CAD build for the part. Positions are in the model's coordinates, mm. A direction names the side the tool comes from. Give positions to 0.01 mm unless a question says otherwise; leave off trailing zeros. Write each loop counter-clockwise with the first axis right and the second up, starting at its lowest first coordinate (ties: lowest second). Pieces come first, ordered by that corner, then holes. Notation, with made-up numbers: (76, 29) - (95, 29) arc R20 ccw to (95, 57) - close; hole circle Ø6 at (-15, 77.25). An arc over 180 degrees is marked (long way). Answer as a JSON object with one key per item and string values.
from build123d import *

# Parameters (mm, degrees)
CUT_EXTRUDE1_DEPTH = 6
CUT_EXTRUDE2_DEPTH = 40


with BuildPart() as part:
    # Sketch1 → Revolve1 (revolve)
    with BuildSketch(Plane.XY):
        with BuildLine():
            Line((8.054036255, 0), (0, 4.65))
            Line((0, 4.65), (0, 11.233))
            Line((0, 11.233), (0.767, 12))
            Line((0.767, 12), (16.233, 12))
            Line((16.233, 12), (17.020818174, 11.212181826))
            ThreePointArc((17.020818174, 11.212181826), (19.144285046, 9.505211333), (21, 11.5))
            Line((21, 11.5), (21, 12.25))
            Line((21, 12.25), (30.021033995, 12.62983301))
            ThreePointArc((30.021033995, 12.62983301), (30.360913423, 12.783353536), (30.5, 13.129390385))
            Line((30.5, 13.129390385), (30.5, 13.175))
            Line((30.5, 13.175), (40, 13.65))
            Line((40, 13.65), (40, 0))
            Line((40, 0), (8.054036255, 0))
        make_face()
    revolve(axis=Axis((40, 0, 0), (-1, 0, 0)))

    # Sketch2 → Cut-Extrude1 (cut)
    with BuildSketch(Plane(origin=(0, 0, 0), x_dir=(0, 0, -1), z_dir=(1, 0, 0))):
        Polygon((-4, -2.309401077), (0, -4.618802154), (4, -2.309401077), (4, 2.309401077), (0, 4.618802154), (-4, 2.309401077), align=None)
    extrude(amount=CUT_EXTRUDE1_DEPTH, mode=Mode.SUBTRACT)

    # Sketch3 → Cut-Revolve1 (revolve, cut)
    with BuildSketch(Plane(origin=(0, 0, 0), x_dir=(1, 0, 0), z_dir=(0, 1, 0))):
        Polygon((6, 0), (6, 4.75), (8, 4.75), (8, 3.5), (10, 3.5), (10, 7.2), (12, 7.2), (12, 7), (42, 7), (42, 0), align=None)
    revolve(axis=Axis((42, 0, 0), (-1, 0, 0)), mode=Mode.SUBTRACT)

    # Sketch4 → Cut-Extrude2 (cut)
    with BuildSketch(Plane(origin=(18, 0, 0), x_dir=(0, 0, -1), z_dir=(1, 0, 0))):
        Polygon((-18.65, 0.5), (-18.65, -0.5), (-0.866025404, -0.5), (-9.758012702, -15.901373781), (-8.891987298, -16.401373781), (0, -1), (8.891987298, -16.401373781), (9.758012702, -15.901373781), (0.866025404, -0.5), (18.65, -0.5), (18.65, 0.5), (0.866025404, 0.5), (9.758012702, 15.901373781), (8.891987298, 16.401373781), (0, 1), (-8.891987298, 16.401373781), (-9.758012702, 15.901373781), (-0.866025404, 0.5), align=None)
    extrude(amount=CUT_EXTRUDE2_DEPTH, mode=Mode.SUBTRACT)


solid = part.part
Item 1: Mould opens along X. For faces 6 (the flat face through (31.29, 8.5, 4.33)), 7 (the flat face through (21, -6, -10)), 8 (the conical face through (35.32, 6.79, -11.57)) say: +X half, -X half, draft (parallel to the pull), parting line (faces both ways), or undercut.
Entries:
{"face 6": "draft", "face 7": "undercut", "face 8": "-X half"}
Item 2: Cut at B-B (x = 33). Give the cut face in (y, z).
Entries:
{"outline": "(-11.76, -6.21) - (-6.3, -3.06) arc R7 cw to (-6.3, 3.06) - (-11.76, 6.21) arc R13.3 ccw to start; (-11.26, -7.08) arc R13.3 ccw to (-0.5, -13.29) - (-0.5, -6.98) arc R7 cw to (-5.8, -3.92) - close; (-11.26, 7.08) - (-5.8, 3.92) arc R7 cw to (-0.5, 6.98) - (-0.5, 13.29) arc R13.3 ccw to start; (0.5, -13.29) arc R13.3 ccw to (11.26, -7.08) - (5.8, -3.92) arc R7 cw to (0.5, -6.98) - close; (0.5, 6.98) arc R7 cw to (5.8, 3.92) - (11.26, 7.08) arc R13.3 ccw to (0.5, 13.29) - close; (6.3, -3.06) - (11.76, -6.21) arc R13.3 ccw to (11.76, 6.21) - (6.3, 3.06) arc R7 cw to start"}
Item 3: Probe line 1 (Y direction, x = 9.4, z = 0); line 2 (Y direction, x = 10.9, z = 0); line 3 (Y direction, x = 37.5, z = -4.75). List the from-to ranges inside material, lowest first. Write a range as from..to.
Entries:
{"line 1": "-12..-3.5, 3.5..12", "line 2": "-12..-7.2, 7.2..12", "line 3": "-12.66..-9.23, -7.23..-5.14, 5.14..7.23, 9.23..12.66"}
Item 4: Cut at D-D (x = 25.5). Give the cut face in (y, z), and give its area (3 significant figures).
Entries:
{"outline": "(-11.01, -5.78) - (-6.3, -3.06) arc R7 cw to (-6.3, 3.06) - (-11.01, 5.78) arc R12.44 ccw to start; (-10.51, -6.65) arc R12.44 ccw to (-0.5, -12.43) - (-0.5, -6.98) arc R7 cw to (-5.8, -3.92) - close; (-10.51, 6.65) - (-5.8, 3.92) arc R7 cw to (-0.5, 6.98) - (-0.5, 12.43) arc R12.44 ccw to start; (0.5, -12.43) arc R12.44 ccw to (10.51, -6.65) - (5.8, -3.92) arc R7 cw to (0.5, -6.98) - close; (0.5, 6.98) arc R7 cw to (5.8, 3.92) - (10.51, 6.65) arc R12.44 ccw to (0.5, 12.43) - close; (6.3, -3.06) - (11.01, -5.78) arc R12.44 ccw to (11.01, 5.78) - (6.3, 3.06) arc R7 cw to start", "area": "300 mm2"}
Item 5: Which spindle directions (+Z, -Z, +X, -X, +Y, -Y) get a long thin tool onto all of the face, cutting with end or side? Do faces 1 (the flat face through (21, -6, 10)), 2 (the flat face through (18, 0, -8)), 3 (the flat face through (31.29, 8.58, -4.376)), 4 (the flat face through (3.65, -3.48, -1.97)), 5 (the cylindrical face through (7.014, 4.214, -2.192)). Say none if no direction does.
Entries:
{"face 1": "+Z, -Y", "face 2": "+Z, -Z, +X", "face 3": "+X", "face 4": "-X", "face 5": "none"}
Item 6: Flat gauge pins, fed straight in: P1, Ø0.8, axis at y = 12.5, z = 1.5, coming from the -X side; P2, Ø5, axis at x = 35.5, y = -2.5, coming from the +Z side; P3, Ø2, axis at x = 25.5, z = 11, coming from the -Y side. Where does each tip first touch, or does it go through?
Entries:
{"P1": "x = 21", "P2": "z = 13.49", "P3": "y = -7.4"}
Item 7: Cut at A-A (x = 4). Give the cut face in (y, z), and give its area (3 significant figures).
Entries:
{"outline": "circle Ø24 at (0, 0); hole (-4.62, 0) - (-2.31, -4) - (2.31, -4) - (4.62, 0) - (2.31, 4) - (-2.31, 4) - close", "area": "397 mm2"}
